from build123d import *

# Parameters (mm, degrees)
F0_W      = 101.6
F0_H      = 12.7
F1_DEPTH  = 25.4
F3_DEPTH  = 25.4
F5_DEPTH  = 25.4
F6_R      = 6.35
F7_DEPTH  = 25.4
F8_R      = 11.983933
F9_DEPTH  = 38.1
F10_R     = 6.35
F11_DEPTH = 50.8
F13_DEPTH = 12.7


with BuildPart() as f1:
    # F0 (on Front) → F1 (new body)
    with BuildSketch(Plane.XZ):
        with Locations((50.8, 6.35)):
            Rectangle(F0_W, F0_H)
    extrude(amount=F1_DEPTH)

    # F2 (on face) → F3 (cut)
    with BuildSketch(Plane.XY.offset(12.7)):
        with BuildLine():
            ThreePointArc((101.6, -12.7), (97.880256, -21.680256), (88.9, -25.4))
            Line((88.9, -25.4), (101.6, -25.4))
            Line((101.6, -25.4), (101.6, -12.7))
        make_face()
        with BuildLine():
            ThreePointArc((88.9, 0), (97.880256, -3.719744), (101.6, -12.7))
            Line((101.6, -12.7), (101.6, 0))
            Line((101.6, 0), (88.9, 0))
        make_face()
    extrude(amount=-F3_DEPTH, mode=Mode.SUBTRACT)

    # F4 (on face) → F5 (cut)
    with BuildSketch(Plane.XY.offset(12.7)):
        with BuildLine():
            ThreePointArc((12.7, -25.4), (3.719744, -21.680256), (0, -12.7))
            Line((0, -12.7), (0, -25.4))
            Line((0, -25.4), (12.7, -25.4))
        make_face()
        with BuildLine():
            ThreePointArc((0, -12.7), (3.719744, -3.719744), (12.7, 0))
            Line((12.7, 0), (0, 0))
            Line((0, 0), (0, -12.7))
        make_face()
    extrude(amount=-F5_DEPTH, mode=Mode.SUBTRACT)

    # F6 (on face) → F7 (cut)
    with BuildSketch(Plane.XY.offset(12.7)):
        with Locations((12.7, -12.7)):
            Circle(F6_R)
    extrude(amount=-F7_DEPTH, mode=Mode.SUBTRACT)

    # F8 (on face) → F9 (join)
    with BuildSketch(Plane.XY.offset(12.7)):
        with Locations((37.383933, -12.7)):
            Circle(F8_R)
    extrude(amount=F9_DEPTH)

    # F10 (on face) → F11 (cut)
    with BuildSketch(Plane.XY.offset(50.8)):
        with Locations((37.383933, -12.7)):
            Circle(F10_R)
    extrude(amount=-F11_DEPTH, mode=Mode.SUBTRACT)

    # F12 (on face) → F13 (cut)
    with BuildSketch(Plane.XY.offset(12.7)):
        with BuildLine():
            ThreePointArc((63.5, -19.05), (67.990128, -17.190128), (69.85, -12.7))
            ThreePointArc((69.85, -12.7), (67.990128, -8.209872), (63.5, -6.35))
            ThreePointArc((63.5, -6.35), (57.15, -12.7), (63.5, -19.05))
        make_face()
        with BuildLine():
            ThreePointArc((63.5, -6.35), (67.990128, -8.209872), (69.85, -12.7))
            ThreePointArc((69.85, -12.7), (67.990128, -17.190128), (63.5, -19.05))
            Line((63.5, -19.05), (88.9, -19.05))
            ThreePointArc((88.9, -19.05), (82.55, -12.7), (88.9, -6.35))
            Line((88.9, -6.35), (63.5, -6.35))
        make_face()
        with BuildLine():
            ThreePointArc((95.25, -12.7), (93.390128, -8.209872), (88.9, -6.35))
            ThreePointArc((88.9, -6.35), (82.55, -12.7), (88.9, -19.05))
            ThreePointArc((88.9, -19.05), (93.390128, -17.190128), (95.25, -12.7))
        make_face()
    extrude(amount=-F13_DEPTH, mode=Mode.SUBTRACT)


solid = f1.part
Geometry check sheet. Reference: the model listing, model coordinates, mm. A direction names the side the tool comes from. Round coordinates to 2 decimals unless told otherwise and drop trailing zeros. Write each loop counter-clockwise with the first axis right and the second up, starting at its lowest first coordinate (ties: lowest second). Pieces come first, ordered by that corner, then holes. Notation, with made-up numbers: (75, 20.25) - (134, 20.25) arc R19 cw to (134, 46.25) - close; hole circle Ø4 at (75.25, 13.25). An arc over 180 degrees is marked (long way). One line per item, written item: value.
1. Depth check by flat-ended pin: pin 1 Ø1.5 at (y, z) = (-21, 20.5) entering from +X; pin 2 Ø6 at (x, z) = (30.5, 27.5) entering from -Y; pin 3 Ø2 at (y, z) = (-18.5, 42) entering from +X. Enter the tip coordinate at first touch or a pass-through.
The answers:
pin 1: stops at x = 46.69
pin 2: stops at y = -24.04
pin 3: stops at x = 48.36
2. Cross-section at D-D on z = 27.5. Record the boundary of the cut face in (x, y).
The answers:
outline: circle Ø23.97 at (37.38, -12.7); hole circle Ø12.7 at (37.38, -12.7)
3. Set-up check for faces 4 (the face through (50, 0, 6)), 5 (the face through (76, -6.35, 6)), 6 (the face through (48.814, -9.1, 31.483)): record each of +Z, -Z, +X, -X, +Y, -Y from which the full face is reachable in a straight line by a thin tool's end or side.
The answers:
face 4: +Z, -Z, +X, -X, +Y
face 5: +Z, -Z
face 6: +Z
4. Cross-section at B-B on z = 11.5. Record the boundary of the cut face in (x, y).
The answers:
outline: (12.7, -25.4) - (88.9, -25.4) arc R12.7 ccw to (88.9, 0) - (12.7, 0) arc R12.7 ccw to start; hole circle Ø12.7 at (12.7, -12.7); hole circle Ø12.7 at (37.38, -12.7); hole (63.5, -19.05) - (88.9, -19.05) arc R6.35 ccw to (88.9, -6.35) - (63.5, -6.35) arc R6.35 ccw to start
5. Scan lines: L1, parallel to Y at x = 12.7, z = 5.75; L2, parallel to Z at x = 5, y = -5.75; L3, parallel to X at y = -16, z = 28.5. Record each from-to range of solid material in increasing order.
The answers:
L1: y = -25.4 to -19.05, -6.35 to 0
L2: z = 0 to 12.7
L3: x = 25.86 to 31.96, 42.81 to 48.9
6. Mould release check, pull along Y, two halves, no side actions. Record for faces 1 (the face through (43, -18, 50.8)), 2 (the face through (36.01, -18.9, 25.76)), 3 (the face through (50, -25.4, 6)): released by +Y, released by -Y, zero draft, split by the parting line, or undercut.
The answers:
face 1: zero draft
face 2: undercut
face 3: released by -Y
7. Cross-section at C-C on y = -15.25. Record the boundary of the cut face in (x, z), and give its area (3 significant figures).
The answers:
outline: (0.26, 0) - (6.88, 0) - (6.88, 12.7) - (0.26, 12.7) - close; (18.52, 0) - (31.57, 0) - (31.57, 50.8) - (25.67, 50.8) - (25.67, 12.7) - (18.52, 12.7) - close; (43.2, 0) - (57.68, 0) - (57.68, 12.7) - (49.09, 12.7) - (49.09, 50.8) - (43.2, 50.8) - close; (94.72, 0) - (101.34, 0) - (101.34, 12.7) - (94.72, 12.7) - close
area: 967 mm^2
8. Cross-section at A-A on x = 68.5. Record the boundary of the cut face in (y, z), and give its area (3 significant figures).
The answers:
outline: (-25.4, 0) - (-19.05, 0) - (-19.05, 12.7) - (-25.4, 12.7) - close; (-6.35, 0) - (0, 0) - (0, 12.7) - (-6.35, 12.7) - close
area: 161 mm^2
